The model under review builds one solid part; all positions refer to its coordinate system, in mm. A direction names the side the tool comes from. Give positions to 0.01 mm unless a question says otherwise; leave off trailing zeros. Write each loop counter-clockwise with the first axis right and the second up, starting at its lowest first coordinate (ties: lowest second). Pieces come first, ordered by that corner, then holes. Notation, with made-up numbers: M 85.5,88.25 L 92.5,88.25 A15 cw 92.5,92.25 Z; hole C -13.5,7 d10. An arc over 180 degrees is marked long. Write each question's results on one line, items separated by ' | '. Start each with the question number.
from build123d import *

# Parameters (mm, degrees)
SKETCH1_W           = 114.3
SKETCH1_H           = 63.5
BOSS_EXTRUDE3_DEPTH = 5.08
SKETCH2_R           = 2.032
CUT_EXTRUDE4_DEPTH  = 131.853148223
CUT_EXTRUDE5_DEPTH  = 131.853148223


with BuildPart() as part:
    # Sketch1 → Boss-Extrude3 (new body)
    with BuildSketch(Plane.XY):
        with Locations((57.15, 31.75)):
            Rectangle(SKETCH1_W, SKETCH1_H)
    extrude(amount=BOSS_EXTRUDE3_DEPTH)

    # Sketch2 → Cut-Extrude4 (cut, through all)
    with BuildSketch(Plane.XY):
        with Locations((88.9, 60.1218)):
            Circle(SKETCH2_R)
        with Locations(Location((88.9, 3.3782, 0), (0, 0, 180))):
            Circle(SKETCH2_R)
        with Locations((25.4, 3.3782)):
            Circle(SKETCH2_R)
        with Locations(Location((25.4, 60.1218, 0), (0, 0, 180))):
            Circle(SKETCH2_R)
        with Locations((10.16, 3.3782)):
            Circle(SKETCH2_R)
        with Locations(Location((10.16, 60.1218, 0), (0, 0, 180))):
            Circle(SKETCH2_R)
        with Locations(Location((104.14, 3.3782, 0), (0, 0, 180))):
            Circle(SKETCH2_R)
        with Locations((104.14, 60.1218)):
            Circle(SKETCH2_R)
    extrude(amount=CUT_EXTRUDE4_DEPTH, mode=Mode.SUBTRACT)

    # Sketch3 → Cut-Extrude5 (cut, through all)
    with BuildSketch(Plane(origin=(0, 0, 0), x_dir=(-1, 0, 0), z_dir=(0, 0, -1))):
        with BuildLine():
            Line((-106.68, 42.164), (-55.88, 42.164))
            ThreePointArc((-55.88, 42.164), (-54.61, 40.894), (-55.88, 39.624))
            Line((-55.88, 39.624), (-106.68, 39.624))
            ThreePointArc((-106.68, 39.624), (-107.95, 40.894), (-106.68, 42.164))
        make_face()
        with BuildLine():
            Line((-106.68, 23.876), (-55.88, 23.876))
            ThreePointArc((-55.88, 23.876), (-54.61, 22.606), (-55.88, 21.336))
            Line((-55.88, 21.336), (-106.68, 21.336))
            ThreePointArc((-106.68, 21.336), (-107.95, 22.606), (-106.68, 23.876))
        make_face()
    extrude(amount=-CUT_EXTRUDE5_DEPTH, mode=Mode.SUBTRACT)


solid = part.part
(1) Machinability: for faces 1 (the cylindrical face through (107.95, 40.87, 2.5)), 2 (the flat face through (0, 31, 3)), which of the approach directions +Z, -Z, +X, -X, +Y, -Y give a long, thin tool a straight path to every point of the face, cutting with its end or side? Answer none if there is none.
(2) Wall thickness on L1, parallel to Y at x = 25.4, z = 1.9; L2, parallel to Y at x = 60, z = 1.1; L3, parallel to Y at x = 88.9, z = 1.25: over which ranges is each line inside the solid? List them lowest first.
(3) Add section B-B (x = 101). State the section outline as (y, z) points, then the cut area to 3 significant figures.
(4) Add section A-A (x = 88.9). State the section outline as (y, z) points, then the cut area to 3 significant figures.
(5) Add section C-C (z = 2.8). Give the number of separate pieces and of enclosed holes in the cut face, then the cut area to 3 significant figures.
(6) Add section D-D (x = 10.16). State the section outline as (y, z) points, then the cut area to 3 significant figures.
Calculated:
1) face 1: +Z, -Z | face 2: +Z, -Z, -X, +Y, -Y
2) L1: y = 0 to 1.35, 5.41 to 58.09, 62.15 to 63.5 | L2: y = 0 to 21.34, 23.88 to 39.62, 42.16 to 63.5 | L3: y = 0 to 1.35, 5.41 to 21.34, 23.88 to 39.62, 42.16 to 58.09, 62.15 to 63.5
3) outline: M 0,0 L 21.34,0 L 21.34,5.08 L 0,5.08 Z; M 23.88,0 L 39.62,0 L 39.62,5.08 L 23.88,5.08 Z; M 42.16,0 L 63.5,0 L 63.5,5.08 L 42.16,5.08 Z | area: 297 mm²
4) outline: M 0,0 L 1.35,0 L 1.35,5.08 L 0,5.08 Z; M 5.41,0 L 21.34,0 L 21.34,5.08 L 5.41,5.08 Z; M 23.88,0 L 39.62,0 L 39.62,5.08 L 23.88,5.08 Z; M 42.16,0 L 58.09,0 L 58.09,5.08 L 42.16,5.08 Z; M 62.15,0 L 63.5,0 L 63.5,5.08 L 62.15,5.08 Z | area: 255 mm²
5) separate pieces: 1 | enclosed holes: 10 | area: 6,890 mm²
6) outline: M 0,0 L 1.35,0 L 1.35,5.08 L 0,5.08 Z; M 5.41,0 L 58.09,0 L 58.09,5.08 L 5.41,5.08 Z; M 62.15,0 L 63.5,0 L 63.5,5.08 L 62.15,5.08 Z | area: 281 mm²
